from build123d import *

# Parameters (mm, degrees)
F0_W     = 12.3
F0_H     = 10.3
F1_DEPTH = 2
F2_DEPTH = 25
F3_R     = 1


with BuildPart() as f1:
    # F0 (on Top) → F1 (new body)
    with BuildSketch(Plane.XY):
        Rectangle(F0_W, F0_H)
        with BuildLine():
            ThreePointArc((1, 2.9), (3.9, 0), (1, -2.9))
            Line((1, -2.9), (-1, -2.9))
            ThreePointArc((-1, -2.9), (-3.9, 0), (-1, 2.9))
            Line((-1, 2.9), (1, 2.9))
        make_face(mode=Mode.SUBTRACT)
    extrude(amount=F1_DEPTH)

    # F0 (on Top) → F2 (join)
    with BuildSketch(Plane.XY):
        with BuildLine():
            Line((-1, -2.9), (1, -2.9))
            ThreePointArc((1, -2.9), (3.9, 0), (1, 2.9))
            Line((1, 2.9), (-1, 2.9))
            ThreePointArc((-1, 2.9), (-3.9, 0), (-1, -2.9))
        make_face()
        with BuildLine():
            ThreePointArc((-1, -1.9), (-2.9, 0), (-1, 1.9))
            Line((-1, 1.9), (1, 1.9))
            ThreePointArc((1, 1.9), (2.9, 0), (1, -1.9))
            Line((1, -1.9), (-1, -1.9))
        make_face(mode=Mode.SUBTRACT)
    extrude(amount=F2_DEPTH)

    # F3
    f3_edges = [f1.edges().sort_by_distance(p)[0] for p in [
        (-3.9, 0, 2),
        (-6.15, 5.15, 1),
        (6.15, 5.15, 1),
        (6.15, -5.15, 1),
        (-6.15, -5.15, 1),
        (2.9, 0, 0),
    ]]
    fillet(f3_edges, radius=F3_R)

    # F5: sweep along a path in F5_path
    with BuildLine(Plane(origin=(-1, 1.9, 25), x_dir=(0, -1, 0), z_dir=(0, 0, -1))) as f5_path:
        Line((0, 0), (0, -2))
        ThreePointArc((0, -2), (1.9, -3.9), (3.8, -2))
        Line((3.8, -2), (3.8, 0))
        ThreePointArc((3.8, 0), (1.9, 1.9), (0, 0))
    # F4 (on Front) → F5 (sweep)
    with BuildSketch(Plane.XZ):
        with BuildLine():
            ThreePointArc((4.3550781059, 28.4958062232), (3.2782925097, 26.8932718666), (2.9, 25))
            Line((2.9, 25), (3.9, 25))
            ThreePointArc((3.9, 25), (4.201510745, 26.5089958069), (5.0597419257, 27.7862648917))
            Line((5.0597419257, 27.7862648917), (4.3550781059, 28.4958062232))
        make_face()
    sweep(path=f5_path.line)


solid = f1.part
CAD build for the part. Positions are in the model's coordinates, mm. A direction names the side the tool comes from. Round coordinates to 2 decimals unless told otherwise and drop trailing zeros. Write each loop counter-clockwise with the first axis right and the second up, starting at its lowest first coordinate (ties: lowest second). Pieces come first, ordered by that corner, then holes. Notation, with made-up numbers: M 5.25,-8 L 59.25,-8 A8 ccw 59.25,7 Z; hole C -32.75,86.25 d5. An arc over 180 degrees is marked long. Put each result on its own line as item: value. Start each with the question number.
1) Drill centre lines: probe 1 along X at (y, z) = (1.5, 25.5); probe 2 along Z at (x, y) = (5.5, -3.75); probe 3 along X at (y, z) = (0.75, 21.25). Where is each one in solid material? Low to high. Write a range as [from, to].
2) Pull direction Z, two halves, no side cores. Call faces 1 (the flat face through (0, 4, 0)), 2 (the cylindrical face through (-5.865, 4.849, 1.014)), 3 (the cylindrical face through (3.9, -0.1, 13.8)), 4 (the conical face through (-4.47, -0.08, 28.38)): pulls with the +Z half, pulls with the -Z half, needs draft (parallel to the pull), parting line crosses it, or undercut.
3) Saw through at B-B, the plane z = 18. Write the cut outline in (x, y), and give its area (3 significant figures).
4) Saw through at A-A, the plane y = 0. Write the cut outline in (x, z), and give its area (3 significant figures).
5) Saw through at C-C, the plane x = -0.25. Write the cut outline in (y, z), and give its area (3 significant figures).
6) 3-axis set-ups, long thin cutter, end or side, ignore diameter. For faces 5 (the cylindrical face through (0.01, 2.29, 26.92)), 6 (the flat face through (0, 1.9, 13)), 7 (the cylindrical face through (-0.01, -3.21, 26.53)): which of +Z, -Z, +X, -X, +Y, -Y reach the whole face in a straight line?
7) Pin check, flat tips, straight feed: pin 1 Ø6 at (x, z) = (-1.5, 11) entering from -Y; pin 2 Ø2 at (x, z) = (0, 11.5) entering from +Y; pin 3 Ø2 at (y, z) = (-3.5, 24) entering from -X. Stop position of each tip, or through.
Resolved:
1. probe 1: [-3.52, -2.21], [2.21, 3.52]
1. probe 2: [0, 2]
1. probe 3: [-3.8, -2.75], [2.75, 3.8]
2. face 1: pulls with the -Z half
2. face 2: needs draft
2. face 3: undercut
2. face 4: pulls with the +Z half
3. outline: M -1,-2.9 L 1,-2.9 A2.9 ccw 1,2.9 L -1,2.9 A2.9 ccw Z; hole M -1,-1.9 L 1,-1.9 A1.9 ccw 1,1.9 L -1,1.9 A1.9 ccw Z
3. area: 19.1 mm²
4. outline: M -6.15,0 L -3.9,0 A1 ccw -2.9,1 L -2.9,25 A4.93 ccw -4.36,28.5 L -5.06,27.79 A3.93 cw -3.9,25 L -3.9,3 A1 cw -4.9,2 L -6.15,2 Z; M 2.9,1 A1 ccw 3.9,0 L 6.15,0 L 6.15,2 L 4.9,2 A1 cw 3.9,3 L 3.9,25 A3.93 cw 5.06,27.79 L 4.36,28.5 A4.93 ccw 2.9,25 Z
4. area: 66.0 mm²
5. outline: M -5.15,0 L -2.9,0 A1 ccw -1.9,1 L -1.9,25 A4.93 ccw -3.36,28.5 L -4.06,27.79 A3.93 cw -2.9,25 L -2.9,3 A1 cw -3.9,2 L -5.15,2 Z; M 1.9,1 A1 ccw 2.9,0 L 5.15,0 L 5.15,2 L 3.9,2 A1 cw 2.9,3 L 2.9,25 A3.93 cw 4.06,27.79 L 3.36,28.5 A4.93 ccw 1.9,25 Z
5. area: 66.0 mm²
6. face 5: +Z
6. face 6: +Z, -Z
6. face 7: +X, -X, -Y
7. pin 1: y = -2.9
7. pin 2: y = 2.9
7. pin 3: x = -2.47
